from build123d import *

# Parameters (mm, degrees)
SKETCH_1_W          = 15
SKETCH_1_H          = 15
SKETCH_1_W_2        = 13
SKETCH_1_H_2        = 13
EXTRUDE_1_DEPTH     = 105
SKETCH_3_R          = 1.5
CUT_EXTRUDE_2_DEPTH = 107.330851591
SKETCH_4_R          = 1.5
CUT_EXTRUDE_3_DEPTH = 107.330851591


with BuildPart() as part:
    # 草图1 → 凸台-拉伸1 (new body)
    with BuildSketch(Plane.XY):
        Rectangle(SKETCH_1_W, SKETCH_1_H)
        Rectangle(SKETCH_1_W_2, SKETCH_1_H_2, mode=Mode.SUBTRACT)
    extrude(amount=EXTRUDE_1_DEPTH)

    # 草图3 → 切除-拉伸2 (cut, through all)
    with BuildSketch(Plane(origin=(0, 7.5, 0), x_dir=(1, 0, 0), z_dir=(0, 1, 0))):
        with Locations(Location((0, -97, 0), (0, 0, 270))):
            Circle(SKETCH_3_R)
        with Locations(Location((0, -89, 0), (0, 0, 270))):
            Circle(SKETCH_3_R)
        with Locations(Location((0, -16, 0), (0, 0, 270))):
            Circle(SKETCH_3_R)
        with Locations(Location((0, -8, 0), (0, 0, 270))):
            Circle(SKETCH_3_R)
    extrude(amount=-CUT_EXTRUDE_2_DEPTH, mode=Mode.SUBTRACT)

    # 草图4 → 切除-拉伸3 (cut, through all)
    with BuildSketch(Plane.ZY.offset(7.5)):
        with Locations((93, 0)):
            Circle(SKETCH_4_R)
        with Locations((83, 0)):
            Circle(SKETCH_4_R)
        with Locations((12, 0)):
            Circle(SKETCH_4_R)
        with Locations((22, 0)):
            Circle(SKETCH_4_R)
    extrude(amount=-CUT_EXTRUDE_3_DEPTH, mode=Mode.SUBTRACT)


solid = part.part
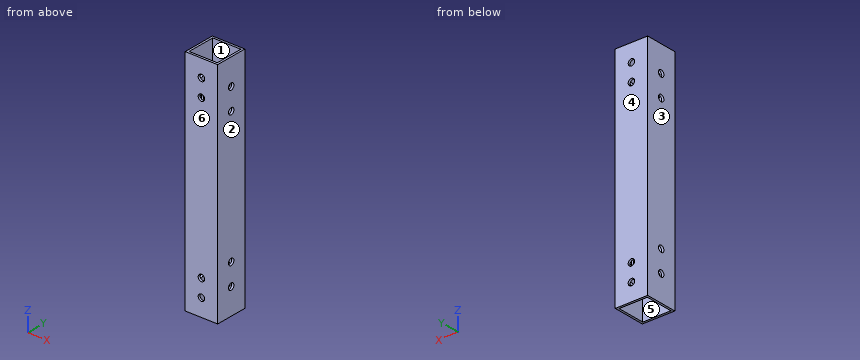
Check sheet for the modelled part. Datum: model origin and axes. Units: mm. Face numbers are marked on the shaded views. A direction names the side the tool comes from. Give positions to 0.01 mm unless a question says otherwise; leave off trailing zeros. Loops run counter-clockwise (first coordinate to the right, second up) from the corner with the lowest first, then second, coordinate; pieces in that order, holes last. Notation, with made-up numbers: M 20.25,-38.75 L 34.25,-38.75 A34 cw 34.25,-3.75 Z; hole C 24,-5.5 d3. An arc over 180 degrees is marked long. Answer as a JSON object with one key per item and string values. Group by question number.
Q1. Access from +Z, -Z, +X, -X, +Y, -Y to the whole of each face (thin tool, end or side, straight path). Record for the marked faces 1 and 2.
Q2. Release check for a two-part mould opening along Y. For the marked faces 3, 4, 5 and 6 record: released by +Y, released by -Y, zero draft, split by the parting line, or undercut.
Q3. Cross-section at C-C on z = 93. Record the cut outline in (x, y), then the cut area to 3 significant figures.
Q4. Material ranges on line 1 along X through (y, z) = (4.25, 17); line 2 along X through (y, z) = (-6.85, 89), recorded low to high. Write a range as [from, to].
Q5. Cross-section at D-D on z = 56. Record the cut outline in (x, y).
Q6. Cross-section at A-A on y = 3. Record the cut outline in (x, z), then the cut area to 3 significant figures.
Evaluation:
{
 "1": {"face 1": "+Z, -Z", "face 2": "+Z, -Z, +X, +Y, -Y"},
 "2": {"face 3": "zero draft", "face 4": "released by +Y", "face 5": "undercut", "face 6": "released by -Y"},
 "3": {"outline": "M -7.5,-7.5 L 7.5,-7.5 L 7.5,-1.5 L 6.5,-1.5 L 6.5,-6.5 L -6.5,-6.5 L -6.5,-1.5 L -7.5,-1.5 Z; M -7.5,1.5 L -6.5,1.5 L -6.5,6.5 L 6.5,6.5 L 6.5,1.5 L 7.5,1.5 L 7.5,7.5 L -7.5,7.5 Z", "area": "50.0 mm2"},
 "4": {"line 1": "x = [-7.5, -6.5], [6.5, 7.5]", "line 2": "x = [-7.5, -1.5], [1.5, 7.5]"},
 "5": {"outline": "M -7.5,-7.5 L 7.5,-7.5 L 7.5,7.5 L -7.5,7.5 Z; hole M -6.5,-6.5 L 6.5,-6.5 L 6.5,6.5 L -6.5,6.5 Z"},
 "6": {"outline": "M -7.5,0 L -6.5,0 L -6.5,105 L -7.5,105 Z; M 6.5,0 L 7.5,0 L 7.5,105 L 6.5,105 Z", "area": "210 mm2"}
}
